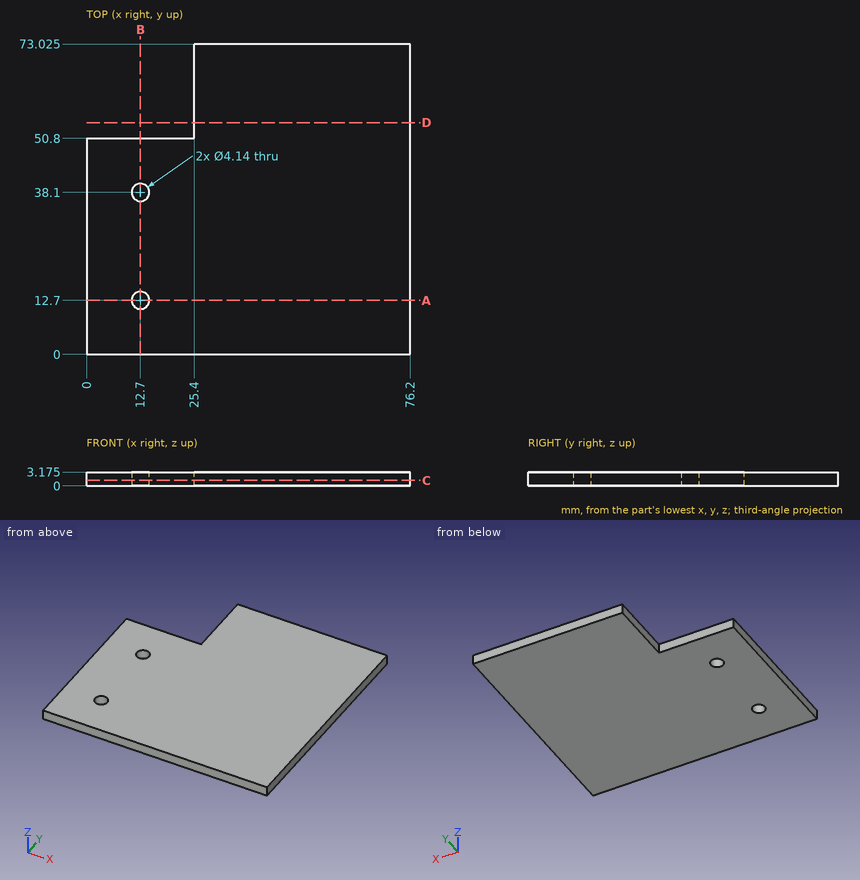
The figure shows three views and two pictorial views of one solid part (mm, origin at its lowest corner). Answer the questions. Coordinates: 2 decimals unless noted, no trailing zeros. Write each loop counter-clockwise with the first axis right and the second up, starting at its lowest first coordinate (ties: lowest second). Pieces come first, ordered by that corner, then holes. Notation, with made-up numbers: (85, 25) -> (140, 25) arc R27 cw to (140, 63) -> close; hole circle Ø11 at (40, 45.25). An arc over 180 degrees is marked (long way). Return JSON: item names as keys, results as strings.
1. A cutting plane is placed at C-C (z = 1.25). Determine the outline of the cut face in (x, y) (1 decimal), and give its area (3 significant figures).
Found:
{"outline": "(0, 0) -> (76.2, 0) -> (76.2, 73) -> (25.4, 73) -> (25.4, 50.8) -> (0, 50.8) -> close; hole circle Ø4.1 at (12.7, 12.7); hole circle Ø4.1 at (12.7, 38.1)", "area": "4,970 mm2"}
2. A cutting plane is placed at D-D (y = 54.5). Determine the outline of the cut face in (x, z) (3 decimals).
Found:
{"outline": "(25.4, 0) -> (76.2, 0) -> (76.2, 3.175) -> (25.4, 3.175) -> close"}
3. A cutting plane is placed at B-B (x = 12.7). Determine the outline of the cut face in (y, z) (1 decimal).
Found:
{"outline": "(0, 0) -> (10.6, 0) -> (10.6, 3.2) -> (0, 3.2) -> close; (14.8, 0) -> (36, 0) -> (36, 3.2) -> (14.8, 3.2) -> close; (40.2, 0) -> (50.8, 0) -> (50.8, 3.2) -> (40.2, 3.2) -> close"}
4. This flat-tipped pin is pushed along its axis until it touches: P1, Ø1, axis at x = 15.5, z = 1.5, coming from the +Y side. Where does it stop, or does it pass through?
Found:
{"P1": "y = 50.8"}
5. Find the intervals of material crossed by line 1 along Y through (x, z) = (12.7, 1.3); line 2 along Y through (x, z) = (19, 2.7); line 3 along X through (y, z) = (68.5, 0.8), in increasing order. Write a range as from..to.
Found:
{"line 1": "0..10.63, 14.77..36.03, 40.17..50.8", "line 2": "0..50.8", "line 3": "25.4..76.2"}
6. A cutting plane is placed at A-A (y = 12.7). Determine the outline of the cut face in (x, z) (1 decimal).
Found:
{"outline": "(0, 0) -> (10.6, 0) -> (10.6, 3.2) -> (0, 3.2) -> close; (14.8, 0) -> (76.2, 0) -> (76.2, 3.2) -> (14.8, 3.2) -> close"}
